Input: part model. Units: mm. Frame: model coordinates. Face numbers are marked on the shaded views. A direction names the side the tool comes from. Coordinates: 2 decimals unless noted, no trailing zeros. Order: outer loops, then holes, each group sorted by start corner. A loop starts at its lowest first (then second) coordinate and runs counter-clockwise, first axis right, second up. Notation, with made-up numbers: (6.25, -29.5) - (32.25, -29.5) arc R32 ccw to (32.25, -2.5) - close; hole circle Ø11 at (10, 75.25). An arc over 180 degrees is marked (long way). Use a Markdown table: item, result. Add a question column.
from build123d import *

# Parameters (mm, degrees)
CUT_EXTRUDE1_DEPTH      = 10
CUT_EXTRUDE1_DEPTH_BACK = 10
SKETCH2_R               = 2.5


with BuildPart() as part:
    # Sketch1 → Revolve1 (revolve)
    with BuildSketch(Plane.XY, mode=Mode.PRIVATE) as revolve1_sk:
        Polygon((0, 0), (0, 5), (40, 5), (40, 12.35), (44.9, 12.35), (44.9, 8.75), (48.1, 8.75), (48.1, 12.35), (53, 12.35), (53, 0), align=None)
    revolve(revolve1_sk.sketch.rotate(Axis((53, 0, 0), (-1, 0, 0)), 90), axis=Axis((53, 0, 0), (-1, 0, 0)))

    # Sketch2 → Cut-Extrude1 (cut, two sides: drawn at the far end of the back side and taken through both)
    with BuildSketch(Plane.XY.offset(-CUT_EXTRUDE1_DEPTH_BACK)):
        with Locations(Location((5, 0, 0), (0, 0, 180))):
            Circle(SKETCH2_R)
    extrude(amount=CUT_EXTRUDE1_DEPTH + CUT_EXTRUDE1_DEPTH_BACK, mode=Mode.SUBTRACT)


solid = part.part
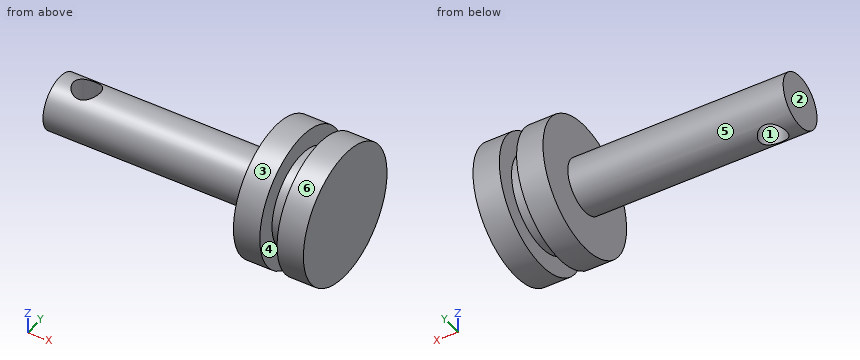
1) Material intervals for L1, parallel to X at y = -9.25, z = 1; L2, parallel to X at y = 5, z = 3; L3, parallel to Y at x = 5, z = -2, sorted ascending.
2) Contact query for flat-ended pins moving along their axis: P1, Ø4, axis at x = 21.5, z = 0.5, coming from the +Y side; P2, Ø1.5, axis at y = -8, z = -5.5, coming from the -X side; P3, Ø10, axis at x = 12.5, z = 7, coming from the +Y side. Output: stop coordinate, or through.
3) Cut plane D-D (x = 5). Return the cut outline in (y, z), and give its area (3 significant figures).
4) Cut plane B-B (z = 0). Return the cut outline in (x, y).
5) Cut plane C-C (z = 6.75). Return the cut outline in (x, y).
6) Pull-direction query (Y, two-part tool) for the marked faces 1, 2 and 3; classes: pulls with the +Y half, pulls with the -Y half, needs draft (parallel to the pull), parting line crosses it, or undercut.
7) Reachability of the marked faces 4, 5 and 6 from +Z, -Z, +X, -X, +Y, -Y: full face, straight path, thin tool, end or side. Return the list, or none.
8) Cut plane A-A (y = 0). Return the cut outline in (x, z), and give its area (3 significant figures).
Computed:
| question | item | result |
|---|---|---|
| 1 | L1 | x = 40 to 44.9, 48.1 to 53 |
| 1 | L2 | x = 40 to 53 |
| 1 | L3 | y = -4.58 to -2.5, 2.5 to 4.58 |
| 2 | P1 | stops at y = 5 |
| 2 | P2 | stops at x = 40 |
| 2 | P3 | stops at y = 4.58 |
| 3 | outline | (-2.5, -4.33) - (-2.5, 4.33) arc R5 ccw to start; (2.5, -4.33) arc R5 ccw to (2.5, 4.33) - close |
| 3 | area | 30.7 mm2 |
| 4 | outline | (0, -5) - (40, -5) - (40, -12.35) - (44.9, -12.35) - (44.9, -8.75) - (48.1, -8.75) - (48.1, -12.35) - (53, -12.35) - (53, 12.35) - (48.1, 12.35) - (48.1, 8.75) - (44.9, 8.75) - (44.9, 12.35) - (40, 12.35) - (40, 5) - (0, 5) - close; hole circle Ø5 at (5, 0) |
| 5 | outline | (40, -10.34) - (44.9, -10.34) - (44.9, -5.57) - (48.1, -5.57) - (48.1, -10.34) - (53, -10.34) - (53, 10.34) - (48.1, 10.34) - (48.1, 5.57) - (44.9, 5.57) - (44.9, 10.34) - (40, 10.34) - close |
| 6 | face 1 | undercut |
| 6 | face 2 | needs draft |
| 6 | face 3 | parting line crosses it |
| 7 | face 4 | none |
| 7 | face 5 | -X |
| 7 | face 6 | +X, -X |
| 8 | outline | (0, -5) - (2.5, -5) - (2.5, 5) - (0, 5) - close; (7.5, -5) - (40, -5) - (40, -12.35) - (44.9, -12.35) - (44.9, -8.75) - (48.1, -8.75) - (48.1, -12.35) - (53, -12.35) - (53, 12.35) - (48.1, 12.35) - (48.1, 8.75) - (44.9, 8.75) - (44.9, 12.35) - (40, 12.35) - (40, 5) - (7.5, 5) - close |
| 8 | area | 648 mm2 |
